The drawing under review shows one solid part. Ordinate dimensions are in mm from its lowest x, y, z. A direction names the side the tool comes from. Round coordinates to 2 decimals unless told otherwise and drop trailing zeros. Use a Markdown table: item, result.
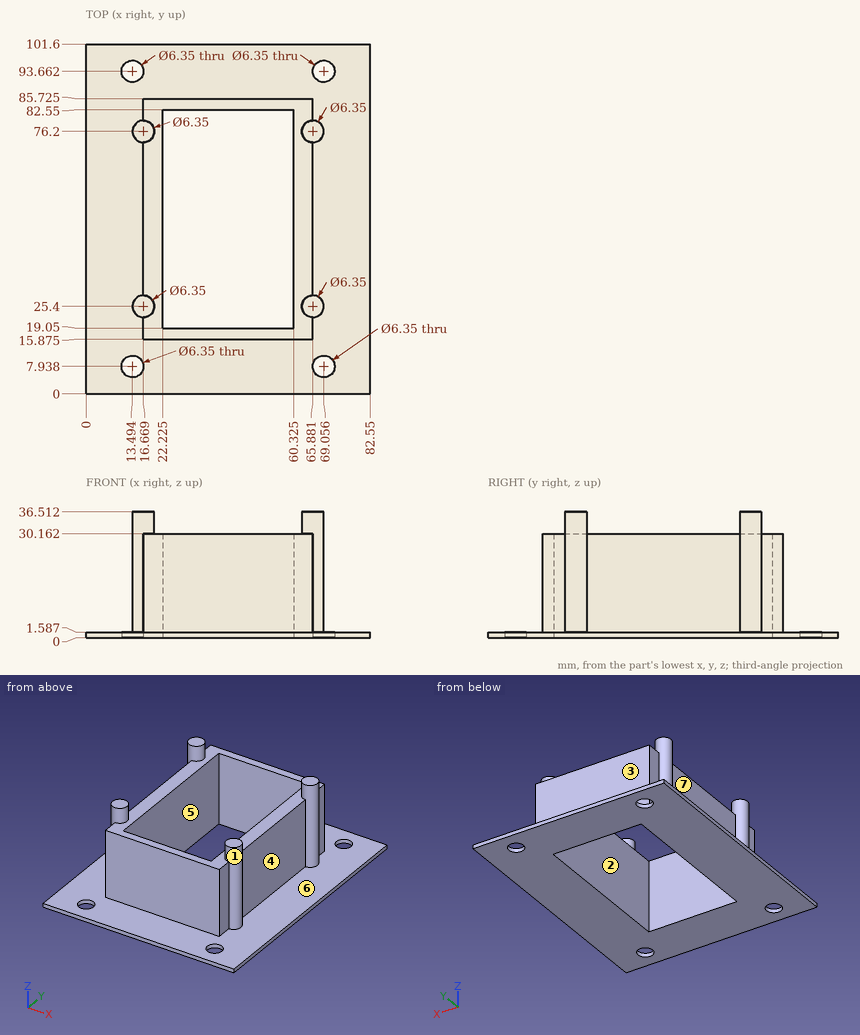
1. The part is to be moulded in two halves that separate along X. For the marked faces 5, 6 and 7, say which applies: pulls with the +X half, pulls with the -X half, needs draft (parallel to the pull), parting line crosses it, or undercut.
Check values:
| item | result |
|---|---|
| face 5 | undercut |
| face 6 | needs draft |
| face 7 | pulls with the -X half |
2. Wall thickness on line 1 along X through (y, z) = (65.5, 26) (1 decimal); line 2 along Y through (x, z) = (16.5, 13); line 3 along Y through (x, z) = (22, 15.5) (1 decimal): over which ranges is each line inside the solid? List them lowest first. Write a range as from..to.
Check values:
| item | result |
|---|---|
| line 1 | x = 16.7..22.2, 60.3..65.9 |
| line 2 | y = 22.23..28.57, 73.03..79.37 |
| line 3 | y = 15.9..85.7 |
3. Machinability: for the marked faces 1, 2, 3 and 4, which of the approach directions +Z, -Z, +X, -X, +Y, -Y give a long, thin tool a straight path to every point of the face, cutting with its end or side? Answer none if there is none.
Check values:
| item | result |
|---|---|
| face 1 | +Z |
| face 2 | +Z, -Z |
| face 3 | +Z, +X, -X, +Y |
| face 4 | +Z, +X |
4. Insertion check: pin 1 (4 mm diameter, centred on x = 45, z = 17.5, fed in from +Y) (1 decimal); pin 2 (9 mm diameter, centred on x = 44.5, z = 17.5, fed in from -Y) (1 decimal); pin 3 (14.5 mm diameter, centred on y = 58, z = 13, fed in from +X). Each pin has a flat end and moves straight along its axis. Give the tip position at first contact, or say it passes through.
Check values:
| item | result |
|---|---|
| pin 1 | stops at y = 85.7 |
| pin 2 | stops at y = 15.9 |
| pin 3 | stops at x = 65.88 |
